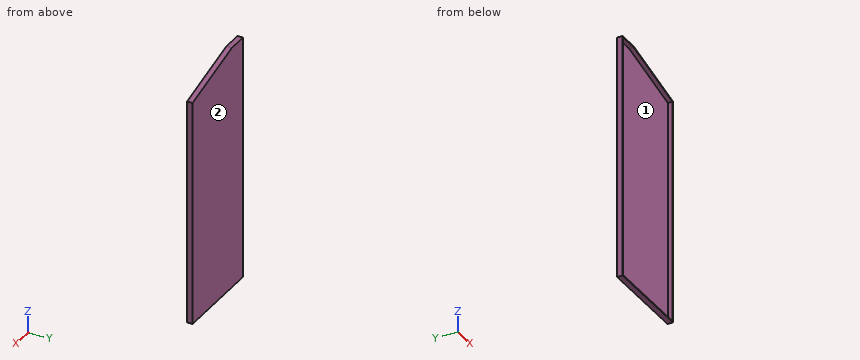
from build123d import *

# Parameters (mm, degrees)
F1_DEPTH = 6.35
F3_DEPTH = 31.75


# Not quite as in the source:
# - a length typed as a fraction of an inch, garbled in the dataset ("3 / 203.2 mm" for 3/8 in), is restored


with BuildPart() as f1:
    # F0 (on Front) → F1 (new body)
    with BuildSketch(Plane.XZ):
        Polygon((0, 1689.1), (0, 0), (635, 0), (635, 1558.925), (139.7, 1689.1), align=None)
    extrude(amount=-F1_DEPTH)

    # F2 (on Front) → F3 (join)
    with BuildSketch(Plane.XZ):
        Polygon((635, 0), (635, 1558.925), (139.7, 1689.1), (0, 1689.1), (0, 0), align=None)
        Polygon((6.35, 6.35), (6.35, 1682.75), (139.7, 1682.75), (628.65, 1554.2439102564), (628.65, 6.35), align=None, mode=Mode.SUBTRACT)
    extrude(amount=F3_DEPTH)


solid = f1.part
Work out the finished part from the listing and answer in its coordinate system (mm). Face numbers are marked on the shaded views. A direction names the side the tool comes from. Round coordinates to 2 decimals unless told otherwise and drop trailing zeros. Order: outer loops, then holes, each group sorted by start corner. A loop starts at its lowest first (then second) coordinate and runs counter-clockwise, first axis right, second up. Notation, with made-up numbers: M 81.5,-9 L 98.5,-9 A30 ccw 98.5,21 Z; hole C 54.25,52 d10. An arc over 180 degrees is marked long. Put each result on its own line as item: value. Start each with the question number.
Q1. Straight lines are drawn through the part: L1, parallel to X at y = -23, z = 1209.5; L2, parallel to Y at x = 471.5, z = 843.5; L3, parallel to Z at x = 112, y = -6. For each, find the intervals that lie inside material, in ascending order. Write a range as [from, to].
Q2. A tool of negligible diameter and unlimited length cuts with its end or side. For the marked faces 1 and 2, from which of +Z, -Z, +X, -X, +Y, -Y can it reach the whole face along a straight path? Write none if from no direction.
Q3. Section B-B, the plane z = 1180 is taken. Write down the section's boundary in (x, y).
Q4. Flat-ended cylindrical pins translate along their axes: pin 1 (4 mm diameter, centred on x = 216, y = -2.5, fed in from +Z); pin 2 (8 mm diameter, centred on x = 505.5, y = -9.5, fed in from +Z). Find the tip coordinate at first contact, or state that the pin passes through.
Q5. Section C-C, the plane x = 223.5 is taken. Write down the section's boundary in (y, z), and give its area (3 significant figures).
Q6. Section A-A, the plane y = -25.5 is taken. Write down the section's boundary in (x, z) (3 decimals), and give its area (3 significant figures).
Findings below:
1. L1: x = [0, 6.35], [628.65, 635]
1. L2: y = [0, 6.35]
1. L3: z = [0, 6.35], [1682.75, 1689.1]
2. face 1: -Y
2. face 2: +Z, -Z, +X, -X, +Y
3. outline: M 0,-31.75 L 6.35,-31.75 L 6.35,0 L 628.65,0 L 628.65,-31.75 L 635,-31.75 L 635,6.35 L 0,6.35 Z
4. pin 1: stops at z = 1669.57
4. pin 2: stops at z = 1594.01
5. outline: M -31.75,0 L 6.35,0 L 6.35,1667.08 L -31.75,1667.08 L -31.75,1660.73 L 0,1660.73 L 0,6.35 L -31.75,6.35 Z
5. area: 11,000 mm^2
6. outline: M 0,0 L 635,0 L 635,1558.925 L 139.7,1689.1 L 0,1689.1 Z; hole M 6.35,6.35 L 628.65,6.35 L 628.65,1554.244 L 139.7,1682.75 L 6.35,1682.75 Z
6. area: 28,500 mm^2
